Source: CAD feature listing. Evaluate the final solid. Frame: model axes, mm. A direction names the side the tool comes from. Give positions to 0.01 mm unless a question says otherwise; leave off trailing zeros. Order: outer loops, then holes, each group sorted by start corner. A loop starts at its lowest first (then second) coordinate and runs counter-clockwise, first axis right, second up. Notation, with made-up numbers: (8.25, -22.75) - (16.25, -22.75) arc R24 cw to (16.25, 4.25) - close; hole circle Ø4 at (83, -31.75). An arc over 180 degrees is marked (long way). Write each question's results on one line, items separated by ' | '. Start each with the question number.
Item 1: Contact query for flat-ended pins moving along their axis: pin 1 Ø0.9 at (x, z) = (-0.5, 1) entering from +Y; pin 2 Ø1.2 at (y, z) = (-4.5, 1) entering from +X; pin 3 Ø6.5 at (x, y) = (4, 3) entering from +Z. Output: stop coordinate, or through.
Item 2: Section C-C on x = 2.5. Output: boundary loops of the cut face in (y, z) (1 decimal).
Item 3: Line query: line 1 along X through (y, z) = (3, 0.55); line 2 along Z through (x, y) = (-12, -13.5); line 3 along X through (y, z) = (4, 0.45). Output: solid intervals per line, ascending.
Item 4: Section A-A on z = 1. Output: boundary loops of the cut face in (x, y) (1 decimal), and give its area (3 significant figures).
Item 5: Set-up query: faces 4 (the flat face through (0, 0, 1.5)), 5 (the flat face through (0, 0, 0)), 6 (the flat face through (7, -3.5, 1)). Return all of +Z, -Z, +X, -X, +Y, -Y with unobstructed straight access to the full face (end or side cutting, diameter ignored); none if empty.
Item 6: Section B-B on y = 0.5. Output: boundary loops of the cut face in (x, z).
Item 7: Mould query, pull axis Y, two halves, no side actions, for faces 1 (the cylindrical face through (-2.737, -12.325, 2.24)), 2 (the flat face through (3.1, -6, 1)), 3 (the flat face through (13, -4, 1.5)). Classes: released by +Y, released by -Y, zero draft, split by the parting line, or undercut.
Item 8: Section D-D on x = -6. Output: boundary loops of the cut face in (y, z).
```python
from build123d import *

# Parameters (mm, degrees)
F0_R     = 19.185
F0_R_2   = 12.625
F1_DEPTH = 1.5
F2_DEPTH = 3
F3_DEPTH = 1.5
F4_DEPTH = 0.4


with BuildPart() as f1:
    # F0 (on Top) → F1 (new body)
    with BuildSketch(Plane.XY):
        Circle(F0_R)
        Circle(F0_R_2, mode=Mode.SUBTRACT)
    extrude(amount=F1_DEPTH)

    # F0 (on Top) → F2 (join)
    with BuildSketch(Plane.XY):
        Circle(F0_R_2)
        with BuildLine():
            ThreePointArc((0, 11.125), (7.866563, 7.866563), (11.125, 0))
            ThreePointArc((11.125, 0), (7.866563, -7.866563), (0, -11.125))
            ThreePointArc((0, -11.125), (-11.125, 0), (0, 11.125))
        make_face(mode=Mode.SUBTRACT)
    extrude(amount=F2_DEPTH)

    # F0 (on Top) → F3 (join)
    with BuildSketch(Plane.XY):
        with BuildLine():
            Line((0, 8.6625), (0, 11.125))
            ThreePointArc((0, 11.125), (-11.125, 0), (0, -11.125))
            Line((0, -11.125), (0, -8.6625))
            Line((0, -8.6625), (-3.1, -8.6625))
            Line((-3.1, -8.6625), (-3.1, -2.4625))
            Line((-3.1, -2.4625), (0, -2.4625))
            Line((0, -2.4625), (0, 2.4625))
            Line((0, 2.4625), (-3.1, 2.4625))
            Line((-3.1, 2.4625), (-3.1, 5.5625))
            Line((-3.1, 5.5625), (-3.1, 8.6625))
            Line((-3.1, 8.6625), (0, 8.6625))
        make_face()
        with BuildLine():
            ThreePointArc((0, -11.125), (7.866563, -7.866563), (11.125, 0))
            ThreePointArc((11.125, 0), (7.866563, 7.866563), (0, 11.125))
            Line((0, 11.125), (0, 8.6625))
            Line((0, 8.6625), (3.1, 8.6625))
            Line((3.1, 8.6625), (3.1, 2.4625))
            Line((3.1, 2.4625), (0, 2.4625))
            Line((0, 2.4625), (0, -2.4625))
            Line((0, -2.4625), (3.1, -2.4625))
            Line((3.1, -2.4625), (3.1, -8.6625))
            Line((3.1, -8.6625), (0, -8.6625))
            Line((0, -8.6625), (0, -11.125))
        make_face()
        Polygon((8.853125, -3.5), (6.953125, -3.5), (5.053125, -3.5), (5.053125, 3.5), (6.953125, 3.5), (8.853125, 3.5), align=None, mode=Mode.SUBTRACT)
    extrude(amount=F3_DEPTH)

    # F0 (on Top) → F4 (join)
    with BuildSketch(Plane.XY):
        with BuildLine():
            Line((3.1, 8.6625), (0, 8.6625))
            Line((0, 8.6625), (0, 8.34375))
            Line((0, 8.34375), (0, 7.4375))
            ThreePointArc((0, 7.4375), (1.325825, 6.888325), (1.875, 5.5625))
            ThreePointArc((1.875, 5.5625), (1.325825, 4.236675), (0, 3.6875))
            Line((0, 3.6875), (0, 2.4625))
            Line((0, 2.4625), (3.1, 2.4625))
            Line((3.1, 2.4625), (3.1, 8.6625))
        make_face()
        with BuildLine():
            Line((0, 8.34375), (0, 8.6625))
            Line((0, 8.6625), (-3.1, 8.6625))
            Line((-3.1, 8.6625), (-3.1, 5.5625))
            Line((-3.1, 5.5625), (-1.875, 5.5625))
            ThreePointArc((-1.875, 5.5625), (-1.325825, 6.888325), (0, 7.4375))
            Line((0, 7.4375), (0, 8.34375))
        make_face()
        with BuildLine():
            Line((-1.875, 5.5625), (-3.1, 5.5625))
            Line((-3.1, 5.5625), (-3.1, 2.4625))
            Line((-3.1, 2.4625), (0, 2.4625))
            Line((0, 2.4625), (0, 3.6875))
            ThreePointArc((0, 3.6875), (-1.325825, 4.236675), (-1.875, 5.5625))
        make_face()
        with BuildLine():
            Line((0, -7.4375), (0, -8.6625))
            Line((0, -8.6625), (3.1, -8.6625))
            Line((3.1, -8.6625), (3.1, -2.4625))
            Line((3.1, -2.4625), (0, -2.4625))
            Line((0, -2.4625), (0, -3.6875))
            ThreePointArc((0, -3.6875), (1.325825, -4.236675), (1.875, -5.5625))
            ThreePointArc((1.875, -5.5625), (1.325825, -6.888325), (0, -7.4375))
        make_face()
        with BuildLine():
            Line((-3.1, -8.6625), (0, -8.6625))
            Line((0, -8.6625), (0, -7.4375))
            ThreePointArc((0, -7.4375), (-1.875, -5.5625), (0, -3.6875))
            Line((0, -3.6875), (0, -2.4625))
            Line((0, -2.4625), (-3.1, -2.4625))
            Line((-3.1, -2.4625), (-3.1, -8.6625))
        make_face()
    extrude(amount=F4_DEPTH)


solid = f1.part
```
Evaluation:
1) pin 1: stops at y = 19.18 | pin 2: stops at x = 18.78 | pin 3: stops at z = 1.5
2) outline: (-19, 0) - (19, 0) - (19, 1.5) - (12.4, 1.5) - (12.4, 3) - (10.8, 3) - (10.8, 1.5) - (8.7, 1.5) - (8.7, 0.4) - (2.5, 0.4) - (2.5, 1.5) - (-2.5, 1.5) - (-2.5, 0.4) - (-8.7, 0.4) - (-8.7, 1.5) - (-10.8, 1.5) - (-10.8, 3) - (-12.4, 3) - (-12.4, 1.5) - (-19, 1.5) - close
3) line 1: x = -18.95 to -3.1, 3.1 to 5.05, 8.85 to 18.95 | line 2: z = 0 to 1.5 | line 3: x = -18.76 to -3.1, 3.1 to 18.76
4) outline: circle Ø38.4 at (0, 0); hole (-3.1, -8.7) - (3.1, -8.7) - (3.1, -2.5) - (-3.1, -2.5) - close; hole (-3.1, 2.5) - (3.1, 2.5) - (3.1, 8.7) - (-3.1, 8.7) - close; hole (5.1, -3.5) - (8.9, -3.5) - (8.9, 3.5) - (5.1, 3.5) - close | area: 1,050 mm^2
5) face 4: +Z | face 5: -Z, +X, -X, +Y, -Y | face 6: +Z, -Z
6) outline: (-19.18, 0) - (5.05, 0) - (5.05, 1.5) - (-11.11, 1.5) - (-11.11, 3) - (-12.62, 3) - (-12.62, 1.5) - (-19.18, 1.5) - close; (8.85, 0) - (19.18, 0) - (19.18, 1.5) - (12.62, 1.5) - (12.62, 3) - (11.11, 3) - (11.11, 1.5) - (8.85, 1.5) - close
7) face 1: split by the parting line | face 2: undercut | face 3: zero draft
8) outline: (-18.22, 0) - (18.22, 0) - (18.22, 1.5) - (11.11, 1.5) - (11.11, 3) - (9.37, 3) - (9.37, 1.5) - (-9.37, 1.5) - (-9.37, 3) - (-11.11, 3) - (-11.11, 1.5) - (-18.22, 1.5) - close
